Work out the finished part from the listing and answer in its coordinate system (mm). Face numbers are marked on the shaded views. Give positions to 0.01 mm unless a question says otherwise; leave off trailing zeros. Order: outer loops, then holes, each group sorted by start corner. A loop starts at its lowest first (then second) coordinate and runs counter-clockwise, first axis right, second up. Notation, with made-up numbers: (18, -1.75) - (47, -1.75) arc R26 ccw to (47, 37.25) - close; hole circle Ø11 at (12.25, 37). An arc over 180 degrees is marked (long way). Put each result on its own line as item: value.
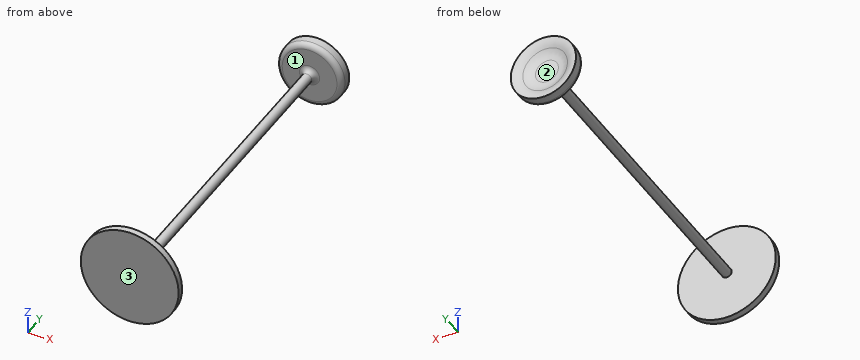
```python
from build123d import *

# Parameters (mm, degrees)
SKETCH1_R           = 75
BOSS_EXTRUDE1_DEPTH = 10
SKETCH2_R           = 7.5
BOSS_EXTRUDE2_DEPTH = 500
SKETCH3_R           = 50
BOSS_EXTRUDE3_DEPTH = 20
FILLET1_R           = 8
SKETCH4_R           = 40.009187759
CUT_EXTRUDE1_DEPTH  = 10
FILLET3_R           = 30
FILLET4_R           = 30


with BuildPart() as part:
    # Sketch1 → Boss-Extrude1 (new body)
    with BuildSketch(Plane(origin=(0, 0, 0), x_dir=(1, 0, 0), z_dir=(0, 1, 0))):
        with Locations(Location((0, 0, 0), (0, 0, 270))):
            Circle(SKETCH1_R)
    extrude(amount=BOSS_EXTRUDE1_DEPTH)

    # Sketch2 → Boss-Extrude2 (add)
    with BuildSketch(Plane(origin=(0, 10, 0), x_dir=(1, 0, 0), z_dir=(0, 1, 0))):
        with Locations(Location((0, 0, 0), (0, 0, 270))):
            Circle(SKETCH2_R)
    extrude(amount=BOSS_EXTRUDE2_DEPTH)

    # Sketch3 → Boss-Extrude3 (add)
    with BuildSketch(Plane(origin=(0, 510, 0), x_dir=(1, 0, 0), z_dir=(0, 1, 0))):
        with Locations(Location((0, 0, 0), (0, 0, 270))):
            Circle(SKETCH3_R)
    extrude(amount=BOSS_EXTRUDE3_DEPTH)

    # Fillet1
    fillet1_edges = [part.edges().sort_by_distance(p)[0] for p in [
        (0, 510, -7.5),
        (0, 510, -50),
    ]]
    fillet(fillet1_edges, radius=FILLET1_R)

    # Sketch4 → Cut-Extrude1 (cut)
    with BuildSketch(Plane(origin=(0, 530, 0), x_dir=(1, 0, 0), z_dir=(0, 1, 0))):
        with Locations(Location((0, 0, 0), (0, 0, 270))):
            Circle(SKETCH4_R)
    extrude(amount=-CUT_EXTRUDE1_DEPTH, mode=Mode.SUBTRACT)

    # Fillet3
    # the kernel refuses this fillet: 30 mm, written as the material it adds along each edge
    with BuildSketch(Plane(origin=(0, 520, 0), x_dir=(0, 0, 1), z_dir=(-1, 0, 0))) as fillet3_piece_1:
        with BuildLine():
            CenterArc((17.648507984, 30), FILLET3_R, 270, 48.189685104)
            Line((17.648507984, 0), (17.648507984, -0.6))
            Line((17.648507984, -0.6), (40.009187759, -0.6))
            Line((40.009187759, -0.6), (40.609187759, 0))
            ThreePointArc((40.609187759, 0), (40.609187759, 5), (40.456401354, 9.6))
            Line((40.456401354, 9.6), (40.009187759, 10))
        make_face()
    revolve(axis=Axis((0, 520, 0), (0, 1, 0)))

    # Fillet4
    # the kernel refuses this fillet: 30 mm, written as the material it takes off along each edge
    with BuildSketch(Plane(origin=(0, 530, 0), x_dir=(0, 0, 1), z_dir=(-1, 0, 0))) as fillet4_piece_1:
        with BuildLine():
            CenterArc((50.832151794, -29.988456502), FILLET4_R, 91.589496733, 31.987749571)
            Line((50, 0), (49.983356964, 0.59976913))
            ThreePointArc((49.983356964, 0.59976913), (45.004593879, 0.6), (40.009187759, 0.6))
            Line((40.009187759, 0.6), (39.561974163, 0.4))
            ThreePointArc((39.561974163, 0.4), (36.891474301, -2.227646014), (33.908493451, -4.494343686))
            Line((33.908493451, -4.494343686), (34.240329889, -4.994228251))
        make_face()
    revolve(axis=Axis((0, 530, 0), (0, 1, 0)), mode=Mode.SUBTRACT)


solid = part.part
```
(1) Section B-B, the plane z = 55 is taken. Write down the section's boundary in (x, y), then the cut area to 3 significant figures.
Geometry check:
outline: (-50.99, 0) - (50.99, 0) - (50.99, 10) - (-50.99, 10) - close
area: 1,020 mm²
(2) Determine the mould class of the marked faces 1, 2 and 3 for opening direction Y: pulls with the +Y half, pulls with the -Y half, needs draft (parallel to the pull), parting line crosses it, or undercut.
Geometry check:
face 1: undercut
face 2: pulls with the +Y half
face 3: pulls with the -Y half
(3) Given pin 1 (12 mm diameter, centred on x = -34, z = -13, fed in from +Y); pin 2 (6 mm diameter, centred on x = -22.5, z = -14, fed in from +Y); pin 3 (10 mm diameter, centred on x = 30.5, z = -30, fed in from +Y), each flat-ended and moving along its own axis, determine where each tip first touches the part or whether it passes through.
Geometry check:
pin 1: stops at y = 528.8
pin 2: stops at y = 522.44
pin 3: stops at y = 529.86
(4) Straight lines are drawn through the part: line 1 (Y direction, x = 63, z = -3.5); line 2 (Y direction, x = -5.5, z = 28); line 3 (X direction, y = 291, z = 6). For each, find the intervals that lie inside material, in ascending order.
Geometry check:
line 1: y = 0 to 10
line 2: y = 0 to 10, 510 to 522.04
line 3: x = -4.5 to 4.5
(5) Section A-A, the plane y = 302 is taken. Write down the section's boundary in (x, z).
Geometry check:
outline: circle Ø15 at (0, 0)
